Design review of the part built by this model. Coordinates are the model's own, in mm. Round coordinates to 2 decimals unless told otherwise and drop trailing zeros. Loops run counter-clockwise (first coordinate to the right, second up) from the corner with the lowest first, then second, coordinate; pieces in that order, holes last. Notation, with made-up numbers: (65, 46) - (97, 46) arc R22 cw to (97, 77) - close; hole circle Ø7 at (-32.5, -36). An arc over 180 degrees is marked (long way). Use one line per item in the form item = value. Start each with the question number.
(1) We need section A-A, the plane x = -64. Write out the cut boundary in (y, z).
(2) Wall thickness on probe 1 along Y at (x, z) = (-78.25, 0); probe 2 along Y at (x, z) = (-40, -17.6); probe 3 along Z at (x, y) = (67, -1.75): over which ranges is each line inside the solid? List them lowest first. Write a range as [from, to].
(3) For pin 1 (1.5 mm diameter, centred on y = -4, z = 0.5, fed in from +X); pin 2 (4 mm diameter, centred on y = -5.5, z = 0, fed in from -X); pin 3 (6 mm diameter, centred on x = -28.5, y = -1, fed in from +Z), all flat-tipped, find the tip position at first contact; note any pin that passes through.
from build123d import *

# Parameters (mm, degrees)
SKETCH_1_W               = 160
SKETCH_1_H               = 40
EXTRUDE_1_DEPTH          = 10
SWEEP_START              = -80
SWEEP_1_DEPTH            = 160
SKETCH_6_R               = 2.575
CUT_EXTRUDE_1_DEPTH      = 3.15
FILLET_1_R               = 5
SKETCH_7_R               = 2.575
CUT_EXTRUDE_2_DEPTH      = 3.15
PATTERN_CIRCULAR_1_COUNT = 2


# Read off the part's stored shape, not the designer's step: Вырез-По траектории1
with BuildPart() as part:
    # Эскиз1 → Бобышка-Вытянуть1 (new body)
    with BuildSketch(Plane(origin=(0, 0, 0), x_dir=(1, 0, 0), z_dir=(0, 1, 0))):
        Rectangle(SKETCH_1_W, SKETCH_1_H)
    extrude(amount=-EXTRUDE_1_DEPTH)

    # Вырез-По траектории1 outline → Вырез-По траектории1 (cut)
    with BuildSketch(Plane.YZ.offset(SWEEP_START)):
        with BuildLine():
            ThreePointArc((0, -18.5), (-1.060660172, -18.939339828), (-1.5, -20))
            Line((-1.5, -20), (0, -20))
            Line((0, -20), (0, -18.5))
        make_face()
    extrude(amount=SWEEP_1_DEPTH, mode=Mode.SUBTRACT)

    # Эскиз6 → Вырез-Вытянуть1 (cut)
    with BuildSketch(Plane(origin=(0, 0, -20), x_dir=(-1, 0, 0), z_dir=(0, 0, -1))):
        with Locations((-40, -5.949176943)):
            Circle(SKETCH_6_R)
        with BuildLine():
            Line((-40, -2.975823057), (-41.2875, -3.719161528))
            ThreePointArc((-41.2875, -3.719161528), (-40, -3.374176943), (-38.7125, -3.719161528))
            Line((-38.7125, -3.719161528), (-40, -2.975823057))
        make_face()
        with Locations((40, -5.949176943)):
            Circle(SKETCH_6_R)
        with BuildLine():
            ThreePointArc((38.7125, -3.719161528), (40, -3.374176943), (41.2875, -3.719161528))
            Line((41.2875, -3.719161528), (40, -2.975823057))
            Line((40, -2.975823057), (38.7125, -3.719161528))
        make_face()
    extrude(amount=-CUT_EXTRUDE_1_DEPTH, mode=Mode.SUBTRACT)

    # Скругление1
    fillet_1_edges = [part.edges().sort_by_distance(p)[0] for p in [
        (0, 0, 20),
    ]]
    fillet(fillet_1_edges, radius=FILLET_1_R)

    # Эскиз7 → Вырез-Вытянуть2 (cut)
    with BuildSketch(Plane.ZY.offset(80)):
        with Locations((0, -5.199176943)):
            Circle(SKETCH_7_R)
        with BuildLine():
            Line((1.2875, -2.969161528), (0, -2.225823057))
            Line((0, -2.225823057), (-1.2875, -2.969161528))
            ThreePointArc((-1.2875, -2.969161528), (0, -2.624176943), (1.2875, -2.969161528))
        make_face()
    cut_extrude_2 = extrude(amount=-CUT_EXTRUDE_2_DEPTH, mode=Mode.SUBTRACT)

    # Круговой массив1: Вырез-Вытянуть2 ×2 about axis
    pattern_circular_1_axis = Axis((0, 0, 0), (0, 1, 0))
    for i in range(1, PATTERN_CIRCULAR_1_COUNT):
        add(cut_extrude_2.rotate(pattern_circular_1_axis, i * 360 / PATTERN_CIRCULAR_1_COUNT), mode=Mode.SUBTRACT)


solid = part.part
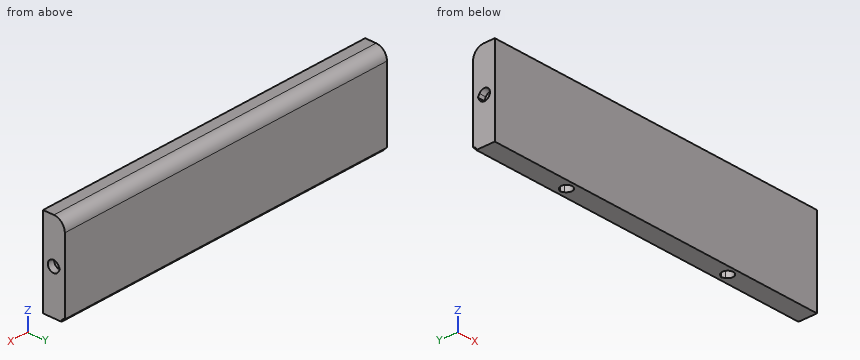
Data:
q1.outline = (-10, -20) - (-1.5, -20) arc R1.5 cw to (0, -18.5) - (0, 15) arc R5 ccw to (-5, 20) - (-10, 20) - close
q2.probe_1 = [-10, -7.77], [-2.23, 0]
q2.probe_2 = [-10, -8.52], [-2.98, 0]
q2.probe_3 = [-20, 18.8]
q3.pin_1 = 76.85
q3.pin_2 = -76.85
q3.pin_3 = 19.9
